Verification items for the finished model (mm, model axes). Round coordinates to 2 decimals unless told otherwise and drop trailing zeros. Loops run counter-clockwise (first coordinate to the right, second up) from the corner with the lowest first, then second, coordinate; pieces in that order, holes last. Notation, with made-up numbers: M -36,-39.5 L -7,-39.5 A33 ccw -7,-9.5 Z; hole C -34.5,-29 d2. An arc over 180 degrees is marked long. Answer as CSV lines item,"result".
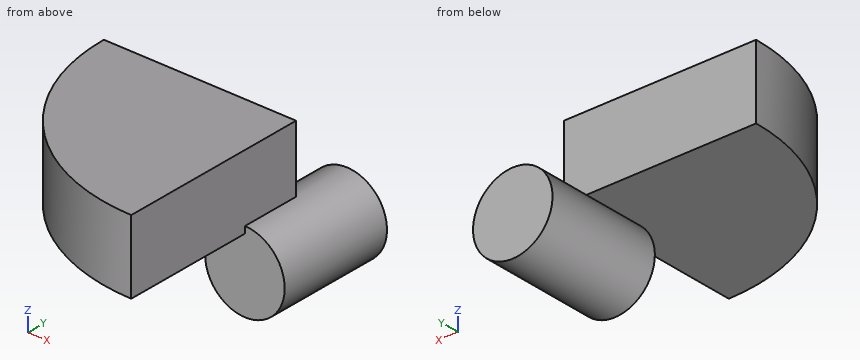
```python
from build123d import *

# Parameters (mm, degrees)
F0_R          = 30
F1_DEPTH      = 90
F3_DEPTH      = 50
F3_DEPTH_BACK = 5


with BuildPart() as f1:
    # F0 (on Front) → F1 (new body)
    with BuildSketch(Plane.XZ):
        with Locations((0, -30)):
            Circle(F0_R)
    extrude(amount=-F1_DEPTH)

    # F2 (on Top) → F3 (join, two sides)
    with BuildSketch(Plane.XY) as f3_sk:
        with BuildLine():
            Line((0, -100), (0, 45))
            Line((0, 45), (-145, 45))
            ThreePointArc((-145, 45), (-102.530483, -57.530483), (0, -100))
        make_face()
    extrude(amount=F3_DEPTH)
    extrude(f3_sk.sketch, amount=-F3_DEPTH_BACK)


solid = f1.part
```
1) Section check C-C (y = -82.5). Record the cut outline in (x, z).
Here are the results:
outline,"M -69.06,-5 L 0,-5 L 0,50 L -69.06,50 Z"
2) Section check B-B (z = -30). Record the cut outline in (x, y).
Here are the results:
outline,"M -30,0 L 30,0 L 30,90 L -30,90 Z"
3) Section check D-D (z = 16). Record the cut outline in (x, y), plus the area to 3 significant figures.
Here are the results:
outline,"M -145,45 A145 ccw 0,-100 L 0,45 Z"
area,"16,500 mm^2"
4) Section check A-A (x = -13.5). Record the cut outline in (y, z), plus the area to 3 significant figures.
Here are the results:
outline,"M -99.37,-5 L 0,-5 L 0,-56.79 L 90,-56.79 L 90,-3.21 L 45,-3.21 L 45,50 L -99.37,50 Z"
area,"12,700 mm^2"
5) Go/stop test with flat-tipped pins: pin 1 (4 mm diameter, centred on y = 28.5, z = -7, fed in from +X); pin 2 (4 mm diameter, centred on x = -82, y = 3.5, fed in from -Z). Record where each tip stops, or that it passes through.
Here are the results:
pin 1,"stops at x = 21.42"
pin 2,"stops at z = -5"
6) Material ranges on probe 1 along Y at (x, z) = (21.5, -39.5); probe 2 along Z at (x, y) = (-80.5, 38); probe 3 along X at (y, z) = (-49, 24.5), recorded low to high.
Here are the results:
probe 1,"y = 0 to 90"
probe 2,"z = -5 to 50"
probe 3,"x = -110.4 to 0"
